Read the model definition and answer for the solid it produces. Units are mm, in the model's axes. Face numbers are marked on the shaded views. A direction names the side the tool comes from. Give positions to 0.01 mm unless a question says otherwise; leave off trailing zeros. Write each loop counter-clockwise with the first axis right and the second up, starting at its lowest first coordinate (ties: lowest second). Pieces come first, ordered by that corner, then holes.
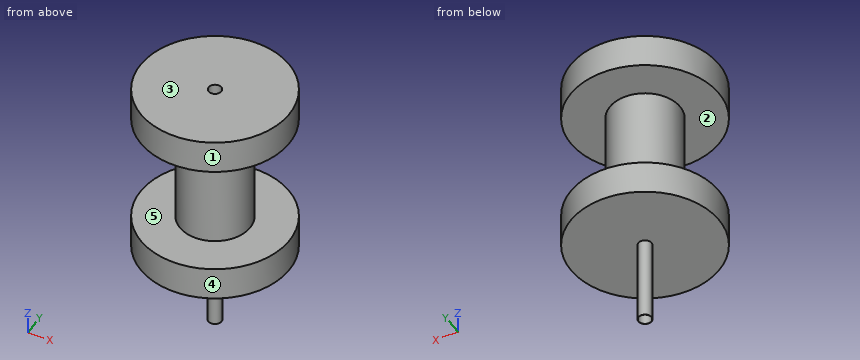
```python
from build123d import *

# Parameters (mm, degrees)
SKETCH1_R            = 1.500124
BOSS_EXTRUDE1_DEPTH  = 29.9974
SHELL3_T             = -0.0508
SKETCH5_R            = 16.891
SKETCH5_R_2          = 1.449324
BOSS_EXTRUDE8_DEPTH  = 7.62
SKETCH6_R            = 7.9999967
SKETCH6_R_2          = 7.62
BOSS_EXTRUDE9_DEPTH  = 25.4
SKETCH7_R            = 16.891
SKETCH7_R_2          = 1.500124
BOSS_EXTRUDE10_DEPTH = 7.62
SKETCH8_R            = 7.9999967
SKETCH8_R_2          = 1.449324
BOSS_EXTRUDE11_DEPTH = 2.54


with BuildPart() as part:
    # Sketch1 → Boss-Extrude1 (new, symmetric)
    with BuildSketch(Plane.XY):
        Circle(SKETCH1_R)
    extrude(amount=BOSS_EXTRUDE1_DEPTH, both=True)

    # Shell3
    shell3_openings = [part.faces().sort_by_distance(p)[0] for p in [
        (0, 0, 29.9974),
        (0, 0, -29.9974),
    ]]
    offset(amount=SHELL3_T, openings=shell3_openings, kind=Kind.INTERSECTION)

    # Sketch5 → Boss-Extrude8 (add)
    with BuildSketch(Plane.XY.offset(29.9974)):
        Circle(SKETCH5_R)
        Circle(SKETCH5_R_2, mode=Mode.SUBTRACT)
    extrude(amount=-BOSS_EXTRUDE8_DEPTH)

    # Sketch6 → Boss-Extrude9 (add)
    with BuildSketch(Plane(origin=(0, 0, 22.3774), x_dir=(-1, 0, 0), z_dir=(0, 0, -1))):
        with Locations(Location((0, 0, 0), (0, 0, 180))):
            Circle(SKETCH6_R)
        Circle(SKETCH6_R_2, mode=Mode.SUBTRACT)
    extrude(amount=BOSS_EXTRUDE9_DEPTH)

    # Sketch7 → Boss-Extrude10 (add)
    with BuildSketch(Plane(origin=(0, 0, -3.0226), x_dir=(-1, 0, 0), z_dir=(0, 0, -1))):
        with Locations(Location((0, 0, 0), (0, 0, 180))):
            Circle(SKETCH7_R)
        Circle(SKETCH7_R_2, mode=Mode.SUBTRACT)
    extrude(amount=BOSS_EXTRUDE10_DEPTH)

    # Sketch8 → Boss-Extrude11 (add)
    with BuildSketch(Plane.XY.offset(29.9974)):
        Circle(SKETCH8_R)
        Circle(SKETCH8_R_2, mode=Mode.SUBTRACT)
    extrude(amount=-BOSS_EXTRUDE11_DEPTH)


solid = part.part
```
Item 1: Which of the six approach directions +Z, -Z, +X, -X, +Y, -Y give full straight-line access (tool end or side, diameter ignored) to the marked faces 1 and 2?
Result set:
face 1: +Z, -Z
face 2: none
Item 2: Determine the mould class of the marked faces 3, 4 and 5 for opening direction Z: pulls with the +Z half, pulls with the -Z half, needs draft (parallel to the pull), parting line crosses it, or undercut.
Result set:
face 3: pulls with the +Z half
face 4: needs draft
face 5: undercut
Item 3: Section A-A (x = 0) is taken. Write down the section's boundary in (y, z).
Result set:
outline: (-16.89, -10.64) - (-1.5, -10.64) - (-1.5, -30) - (-1.45, -30) - (-1.45, 30) - (-16.89, 30) - (-16.89, 22.38) - (-8, 22.38) - (-8, -3.02) - (-16.89, -3.02) - close; (1.45, -30) - (1.5, -30) - (1.5, -10.64) - (16.89, -10.64) - (16.89, -3.02) - (8, -3.02) - (8, 22.38) - (16.89, 22.38) - (16.89, 30) - (1.45, 30) - close; hole (-7.62, -3.02) - (-1.5, -3.02) - (-1.5, 22.38) - (-7.62, 22.38) - close; hole (1.5, -3.02) - (7.62, -3.02) - (7.62, 22.38) - (1.5, 22.38) - close
Item 4: Section D-D (y = 10.5) is taken. Write down the section's boundary in (x, z), and give its area (3 significant figures).
Result set:
outline: (-13.23, -10.64) - (13.23, -10.64) - (13.23, -3.02) - (-13.23, -3.02) - close; (-13.23, 22.38) - (13.23, 22.38) - (13.23, 30) - (-13.23, 30) - close
area: 403 mm2
Item 5: Each of these flat-tipped pins is pushed along its axis until it touches: pin 1 Ø3 at (x, z) = (-4.5, 18) entering from +Y; pin 2 Ø5 at (x, z) = (-2, -5.5) entering from -Y; pin 3 Ø12 at (x, z) = (2.5, 14.5) entering from -Y; pin 4 Ø5 at (y, z) = (1, 13.5) entering from -X. Where does it stop, or does it pass through?
Result set:
pin 1: stops at y = 7.42
pin 2: stops at y = -16.89
pin 3: stops at y = -8
pin 4: stops at x = -8
Item 6: Find the intervals of material crossed by line 1 along Z through (x, y) = (-3.5, 9); line 2 along Y through (x, z) = (6.5, 20.5); line 3 along Y through (x, z) = (7, -1), in increasing order.
Result set:
line 1: z = -10.64 to -3.02, 22.38 to 30
line 2: y = -4.66 to -3.98, 3.98 to 4.66
line 3: y = -3.87 to -3.01, 3.01 to 3.87
Item 7: Section C-C (z = 9) is taken. Write down the section's boundary in (x, y).
Result set:
outline: circle Ø16 at (0, 0); circle Ø3 at (0, 0); hole circle Ø15.24 at (0, 0); hole circle Ø2.9 at (0, 0)
